The figure shows three views and two pictorial views of one solid part (mm, origin at its lowest corner). Answer the questions. Give positions to 0.01 mm unless a question says otherwise; leave off trailing zeros. Write each loop counter-clockwise with the first axis right and the second up, starting at its lowest first coordinate (ties: lowest second). Pieces come first, ordered by that corner, then holes. Notation, with made-up numbers: (88.25, -9) -> (119.25, -9) arc R29 cw to (119.25, 25) -> close; hole circle Ø1 at (-23.5, -1). An arc over 180 degrees is marked (long way). Use a Markdown table: item, result.
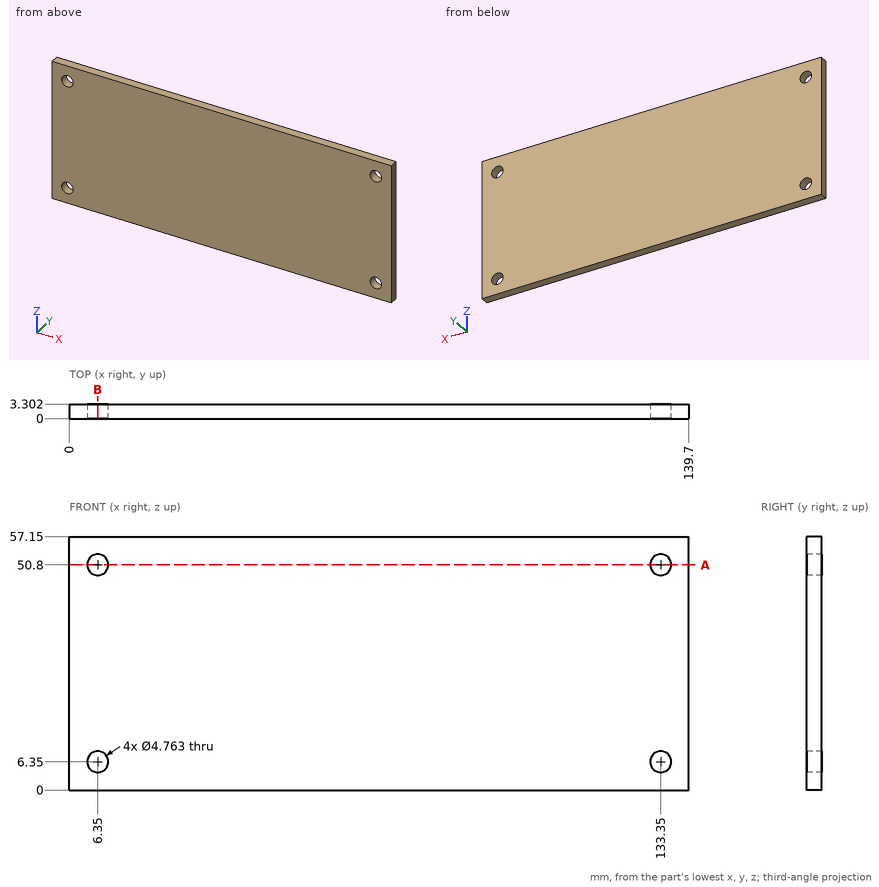
Item 1: A cutting plane is placed at A-A (z = 50.8). Give the vertices of the cut face in (x, y).
Return value:
| item | result |
|---|---|
| outline | (0, 0) -> (3.97, 0) -> (3.97, 3.3) -> (0, 3.3) -> close; (8.73, 0) -> (130.97, 0) -> (130.97, 3.3) -> (8.73, 3.3) -> close; (135.73, 0) -> (139.7, 0) -> (139.7, 3.3) -> (135.73, 3.3) -> close |
Item 2: Straight lines are drawn through the part: line 1 along X through (y, z) = (0.2, 6.5); line 2 along Z through (x, y) = (133.35, 0.7); line 3 along X through (y, z) = (2.35, 5). For each, find the intervals that lie inside material, in ascending order. Write a range as [from, to].
Return value:
| item | result |
|---|---|
| line 1 | [0, 3.97], [8.73, 130.97], [135.73, 139.7] |
| line 2 | [0, 3.97], [8.73, 48.42], [53.18, 57.15] |
| line 3 | [0, 4.39], [8.31, 131.39], [135.31, 139.7] |
Item 3: A cutting plane is placed at B-B (x = 6.35). Give the vertices of the cut face in (y, z).
Return value:
| item | result |
|---|---|
| outline | (0, 0) -> (3.3, 0) -> (3.3, 3.97) -> (0, 3.97) -> close; (0, 8.73) -> (3.3, 8.73) -> (3.3, 48.42) -> (0, 48.42) -> close; (0, 53.18) -> (3.3, 53.18) -> (3.3, 57.15) -> (0, 57.15) -> close |
